Geometry check sheet. Reference: the model listing, model coordinates, mm. Face numbers are marked on the shaded views. A direction names the side the tool comes from. Coordinates: 2 decimals unless noted, no trailing zeros. Loops run counter-clockwise (first coordinate to the right, second up) from the corner with the lowest first, then second, coordinate; pieces in that order, holes last. Notation, with made-up numbers: M 48.5,-0.75 L 70.5,-0.75 A15 cw 70.5,25.25 Z; hole C 56,1.5 d10. An arc over 180 degrees is marked long. Use CSV: the item, a comma, the result in double quotes.
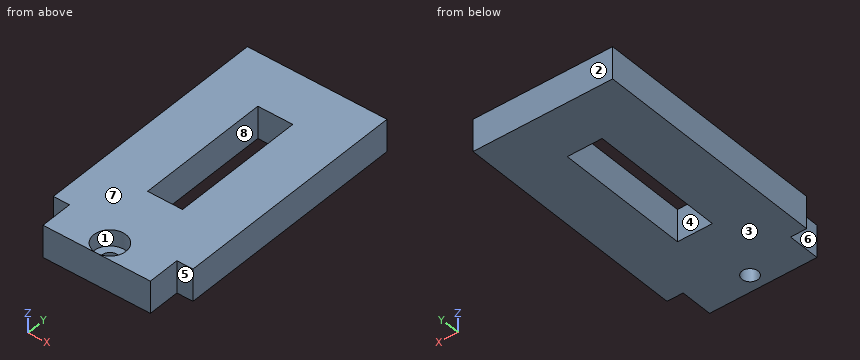
```python
from build123d import *

# Parameters (mm, degrees)
ESQUISSE1_W             = 44
ESQUISSE1_H             = 44
BOSS_EXTRU_1_DEPTH      = 6
ESQUISSE2_W             = 20
ESQUISSE2_H             = 6
BOSS_EXTRU_3_DEPTH      = 6
ESQUISSE3_W             = 6.5
ESQUISSE3_H             = 25
ENL_V_MAT_EXTRU_1_DEPTH = 6
ESQUISSE4_W             = 9
ESQUISSE4_H             = 44
ENL_V_MAT_EXTRU_2_DEPTH = 6
ESQUISSE5_R             = 1.5
ENL_V_MAT_EXTRU_3_DEPTH = 6
ESQUISSE6_R             = 2.995
ENL_V_MAT_EXTRU_4_DEPTH = 3


with BuildPart() as part:
    # Esquisse1 → Boss.-Extru.1 (new body)
    with BuildSketch(Plane.XY):
        with Locations((22, 22)):
            Rectangle(ESQUISSE1_W, ESQUISSE1_H)
    extrude(amount=BOSS_EXTRU_1_DEPTH)

    # Esquisse2 → Boss.-Extru.3 (add)
    with BuildSketch(Plane.XY.offset(6)):
        with Locations((22, -3)):
            Rectangle(ESQUISSE2_W, ESQUISSE2_H)
    extrude(amount=-BOSS_EXTRU_3_DEPTH)

    # Esquisse3 → Enlèv. mat.-Extru.1 (cut)
    with BuildSketch(Plane.XY.offset(6)):
        with Locations((22, 22)):
            Rectangle(ESQUISSE3_W, ESQUISSE3_H)
    extrude(amount=-ENL_V_MAT_EXTRU_1_DEPTH, mode=Mode.SUBTRACT)

    # Esquisse4 → Enlèv. mat.-Extru.2 (cut)
    with BuildSketch(Plane.XY.offset(6)):
        with Locations((4.5, 22)):
            Rectangle(ESQUISSE4_W, ESQUISSE4_H)
        with Locations((39.5, 22)):
            Rectangle(ESQUISSE4_W, ESQUISSE4_H)
    extrude(amount=-ENL_V_MAT_EXTRU_2_DEPTH, mode=Mode.SUBTRACT)

    # Esquisse5 → Enlèv. mat.-Extru.3 (cut)
    with BuildSketch(Plane.XY.offset(6)):
        with Locations((22, -3)):
            Circle(ESQUISSE5_R)
    extrude(amount=-ENL_V_MAT_EXTRU_3_DEPTH, mode=Mode.SUBTRACT)

    # Esquisse6 → Enlèv. mat.-Extru.4 (cut)
    with BuildSketch(Plane.XY.offset(6)):
        with Locations((22, -3)):
            Circle(ESQUISSE6_R)
    extrude(amount=-ENL_V_MAT_EXTRU_4_DEPTH, mode=Mode.SUBTRACT)


solid = part.part
```
1. Section check A-A, the plane y = 26. Record the cut outline in (x, z).
The answers:
outline,"M 9,0 L 18.75,0 L 18.75,6 L 9,6 Z; M 25.25,0 L 35,0 L 35,6 L 25.25,6 Z"
2. Release check for a two-part mould opening along Y. For the marked faces 1, 2, 3 and 4 record: +Y half, -Y half, draft (parallel to the pull), parting line (faces both ways), or undercut.
The answers:
face 1,"undercut"
face 2,"+Y half"
face 3,"draft"
face 4,"undercut"
3. Section check D-D, the plane y = -3. Record the cut outline in (x, z) (3 decimals), plus the area to 3 significant figures.
The answers:
outline,"M 12,0 L 20.5,0 L 20.5,3 L 19.005,3 L 19.005,6 L 12,6 Z; M 23.5,0 L 32,0 L 32,6 L 24.995,6 L 24.995,3 L 23.5,3 Z"
area,"93.0 mm^2"
4. Set-up check for the marked faces 5, 6, 7 and 8: record each of +Z, -Z, +X, -X, +Y, -Y from which the full face is reachable in a straight line by a thin tool's end or side.
The answers:
face 5,"+Z, -Z, +X, -Y"
face 6,"+Z, -Z, -X, -Y"
face 7,"+Z, +X, -X, +Y, -Y"
face 8,"+Z, -Z"
5. Section check B-B, the plane z = 4.5. Record the cut outline in (x, y) (3 decimals), plus the area to 3 significant figures.
The answers:
outline,"M 9,0 L 12,0 L 12,-6 L 32,-6 L 32,0 L 35,0 L 35,44 L 9,44 Z; hole M 18.75,9.5 L 25.25,9.5 L 25.25,34.5 L 18.75,34.5 Z; hole C 22,-3 d5.99"
area,"1,070 mm^2"
6. Thickness scan on line 1 (Y direction, x = 22, z = 2.1); line 2 (X direction, y = 34, z = 5.7); line 3 (Y direction, x = 25, z = 1). Record the ranges inside material, lowest first. Write a range as [from, to].
The answers:
line 1,"[-6, -4.5], [-1.5, 9.5], [34.5, 44]"
line 2,"[9, 18.75], [25.25, 35]"
line 3,"[-6, 9.5], [34.5, 44]"
7. Gauge pin test, flat ends, axial feed: P1, Ø1.5, axis at x = 34, z = 3, coming from the -Y side; P2, Ø5, axis at x = 22, y = -3, coming from the +Z side. Record the tip position at first contact, or that the pin passes through.
The answers:
P1,"y = 0"
P2,"z = 3"
8. Section check C-C, the plane x = 22. Record the cut outline in (y, z) (3 decimals).
The answers:
outline,"M -6,0 L -4.5,0 L -4.5,3 L -5.995,3 L -5.995,6 L -6,6 Z; M -1.5,0 L 9.5,0 L 9.5,6 L -0.005,6 L -0.005,3 L -1.5,3 Z; M 34.5,0 L 44,0 L 44,6 L 34.5,6 Z"
